```python
from build123d import *

# Parameters (mm, degrees)
SKETCH1_W           = 206
SKETCH1_H           = 176
BOSS_EXTRUDE1_DEPTH = 2
FILLET1_R           = 10
SKETCH2_R           = 2
CUT_EXTRUDE1_DEPTH  = 5
SKETCH3_R           = 7.6
SKETCH3_R_2         = 10
CUT_EXTRUDE2_DEPTH  = 5
SKETCH4_W           = 83.45
SKETCH4_H           = 100
CUT_EXTRUDE3_DEPTH  = 10


with BuildPart() as part:
    # Sketch1 → Boss-Extrude1 (new body)
    with BuildSketch(Plane.XY):
        with Locations((103, -88)):
            Rectangle(SKETCH1_W, SKETCH1_H)
    extrude(amount=BOSS_EXTRUDE1_DEPTH)

    # Fillet1
    fillet1_edges = [part.edges().sort_by_distance(p)[0] for p in [
        (0, 0, 1),
        (206, 0, 1),
        (206, -176, 1),
        (0, -176, 1),
    ]]
    fillet(fillet1_edges, radius=FILLET1_R)

    # Sketch2 → Cut-Extrude1 (cut)
    with BuildSketch(Plane(origin=(0, 0, 0), x_dir=(-1, 0, 0), z_dir=(0, 0, -1))):
        with Locations((-198.78553391, -7.21446609)):
            Circle(SKETCH2_R)
        with Locations((-7.21446609, -7.21446609)):
            Circle(SKETCH2_R)
        with Locations((-7.21446609, -168.78553391)):
            Circle(SKETCH2_R)
        with Locations((-198.78553391, -168.78553391)):
            Circle(SKETCH2_R)
    extrude(amount=-CUT_EXTRUDE1_DEPTH, mode=Mode.SUBTRACT)

    # Sketch3 → Cut-Extrude2 (cut)
    with BuildSketch(Plane(origin=(0, 0, 0), x_dir=(-1, 0, 0), z_dir=(0, 0, -1))):
        with Locations((-103, -14)):
            Circle(SKETCH3_R)
        with Locations((-129.5, -42)):
            Circle(SKETCH3_R_2)
        with Locations((-103, -42)):
            Circle(SKETCH3_R)
        with Locations((-76.5, -42)):
            Circle(SKETCH3_R_2)
    extrude(amount=-CUT_EXTRUDE2_DEPTH, mode=Mode.SUBTRACT)

    # Sketch4 → Cut-Extrude3 (cut)
    with BuildSketch(Plane.XY.offset(2)):
        with Locations((61.275, -109.5)):
            Rectangle(SKETCH4_W, SKETCH4_H)
        with Locations((144.725, -109.5)):
            Rectangle(SKETCH4_W, SKETCH4_H)
    extrude(amount=-CUT_EXTRUDE3_DEPTH, mode=Mode.SUBTRACT)


solid = part.part
```
Input: part model. Units: mm. Frame: model coordinates. Round coordinates to 2 decimals unless told otherwise and drop trailing zeros. Order: outer loops, then holes, each group sorted by start corner. A loop starts at its lowest first (then second) coordinate and runs counter-clockwise, first axis right, second up. Notation, with made-up numbers: (-38, 6.25) - (-4, 6.25) arc R13 cw to (-4, 28.25) - close; hole circle Ø2 at (10, 37.5). An arc over 180 degrees is marked (long way). Answer in a Markdown table with one row per item.
Item 1: Pin query (flat end, axial travel): pin 1 (12 mm diameter, centred on x = 103, y = -42, fed in from -Z). Return the tip coordinate at first contact, or that it passes through.
Model answer:
| item | result |
|---|---|
| pin 1 | passes through |
Item 2: Section query D-D (x = 36). Return the cut outline in (y, z), then the cut area to 3 significant figures.
Model answer:
| item | result |
|---|---|
| outline | (-176, 0) - (-159.5, 0) - (-159.5, 2) - (-176, 2) - close; (-59.5, 0) - (0, 0) - (0, 2) - (-59.5, 2) - close |
| area | 152 mm² |
Item 3: Mould query, pull axis X, two halves, no side actions, for faces 1 (the cylindrical face through (2.85, -172.99, 1.01)), 2 (the cylindrical face through (137.44, -48.08, 0.99)), 3 (the cylindrical face through (203.15, -3.01, 1.01)), 4 (the flat face through (102, -28, 2)). Classes: released by +X, released by -X, zero draft, split by the parting line, or undercut.
Model answer:
| item | result |
|---|---|
| face 1 | released by -X |
| face 2 | undercut |
| face 3 | released by +X |
| face 4 | zero draft |
Item 4: Section query B-B (y = -139.5). Return the cut outline in (x, z), then the cut area to 3 significant figures.
Model answer:
| item | result |
|---|---|
| outline | (0, 0) - (19.55, 0) - (19.55, 2) - (0, 2) - close; (186.45, 0) - (206, 0) - (206, 2) - (186.45, 2) - close |
| area | 78.2 mm² |
Item 5: Line query: line 1 (Y direction, x = 64, z = 0.95); line 2 (X direction, y = -95, z = 1.55); line 3 (Y direction, x = 133, z = 1.55). Output: solid intervals per line, ascending.
Model answer:
| item | result |
|---|---|
| line 1 | y = -176 to -159.5, -59.5 to 0 |
| line 2 | x = 0 to 19.55, 186.45 to 206 |
| line 3 | y = -176 to -159.5, -59.5 to -51.37, -32.63 to 0 |
Item 6: Section query C-C (x = 103). Return the cut outline in (y, z), then the cut area to 3 significant figures.
Model answer:
| item | result |
|---|---|
| outline | (-176, 0) - (-159.5, 0) - (-159.5, 2) - (-176, 2) - close; (-59.5, 0) - (-49.6, 0) - (-49.6, 2) - (-59.5, 2) - close; (-34.4, 0) - (-21.6, 0) - (-21.6, 2) - (-34.4, 2) - close; (-6.4, 0) - (0, 0) - (0, 2) - (-6.4, 2) - close |
| area | 91.2 mm² |
Item 7: Section query A-A (x = 129.5). Return the cut outline in (y, z).
Model answer:
| item | result |
|---|---|
| outline | (-176, 0) - (-159.5, 0) - (-159.5, 2) - (-176, 2) - close; (-59.5, 0) - (-52, 0) - (-52, 2) - (-59.5, 2) - close; (-32, 0) - (0, 0) - (0, 2) - (-32, 2) - close |
